Read the model definition and answer for the solid it produces. Units are mm, in the model's axes. A direction names the side the tool comes from. Coordinates: 2 decimals unless noted, no trailing zeros. Loops run counter-clockwise (first coordinate to the right, second up) from the corner with the lowest first, then second, coordinate; pieces in that order, holes last.
Q1. Section B-B (z = 3.9) is taken. Count the separate pieces of the cut face and the enclosed holes in it, then the cut area to 3 significant figures.
Q2. Section A-A (y = 0) is taken. Give the vertices of the cut face in (x, z), then the cut area to 3 significant figures.
Q3. Section C-C (x = 35) is taken. Give the vertices of the cut face in (y, z).
Q4. Which of the six approach directions +Z, -Z, +X, -X, +Y, -Y give full straight-line access (tool end or side, diameter ignored) to faces 1 (the face through (1, 19, 5)), 2 (the face through (69, -31, 3))?
Q5. The mould has two halves that part along Y. Classify faces 3 (the face through (1, -69.382, 2)), 4 (the face through (-3.37, 104.946, 2.465)), 5 (the face through (1, 19, 0)), 6 (the face through (70.87, -39.84, 2.54)): pulls with the +Y half, pulls with the -Y half, needs draft (parallel to the pull), parting line crosses it, or undercut.
Q6. Straight lines are drawn through the part: line 1 (Y direction, x = 0, z = 2.8); line 2 (X direction, y = -44, z = 4); line 3 (Y direction, x = 28, z = 2.5). For each, find the intervals that lie inside material, in ascending order.
Q7. Section D-D (y = 45.5) is taken. Give the vertices of the cut face in (x, z), then the cut area to 3 significant figures.
Q8. Flat-ended cylindrical pins translate along their axes: P1, Ø1.6, axis at x = 28, y = -28, coming from the +Z side; P2, Ø5, axis at x = 0, y = 102.5, coming from the +Z side; P3, Ø1.1, axis at x = 26, z = 2, coming from the +Y side; P4, Ø1.5, axis at y = -3.5, z = 2.5, coming from the -X side. Find the tip coordinate at first contact, or state that the pin passes through.
from build123d import *

# Parameters (mm, degrees)
BOSS_EXTRU_1_DEPTH      = 5
ESQUISSE2_R             = 1.5
ENL_V_MAT_EXTRU_1_DEPTH = 5
ESQUISSE3_R             = 1
ENL_V_MAT_EXTRU_2_DEPTH = 149.576579581
ENL_V_MAT_EXTRU_3_DEPTH = 149.576579581
ESQUISSE5_W             = 3.649999998
ESQUISSE5_H             = 20
ENL_V_MAT_EXTRU_4_DEPTH = 149.576579581


with BuildPart() as part:
    # Esquisse1 → Boss.-Extru.1 (new body)
    with BuildSketch(Plane.XY):
        with BuildLine():
            Line((78.81072608, -69.38205427), (-78.81072608, -69.38205427))
            ThreePointArc((-78.81072608, -69.38205427), (0, 105), (78.81072608, -69.38205427))
        make_face()
    extrude(amount=BOSS_EXTRU_1_DEPTH)

    # Esquisse2 → Enlèv. mat.-Extru.1 (cut)
    with BuildSketch(Plane.XY.offset(5)):
        with Locations((0, 102.5)):
            Circle(ESQUISSE2_R)
        with Locations((72.478445072, 72.478445072)):
            Circle(ESQUISSE2_R)
        with Locations((-72.478445072, 72.478445072)):
            Circle(ESQUISSE2_R)
    extrude(amount=-ENL_V_MAT_EXTRU_1_DEPTH, mode=Mode.SUBTRACT)

    # Esquisse3 → Enlèv. mat.-Extru.2 (cut, through all)
    with BuildSketch(Plane.XY.offset(5)):
        with Locations((20.000000004, 41.999999998)):
            Circle(ESQUISSE3_R)
        with Locations((-19.999999996, 42.000000002)):
            Circle(ESQUISSE3_R)
        with Locations((-28.000000003, -27.999999997)):
            Circle(ESQUISSE3_R)
        with Locations((27.999999997, -28.000000003)):
            Circle(ESQUISSE3_R)
    extrude(amount=-ENL_V_MAT_EXTRU_2_DEPTH, mode=Mode.SUBTRACT)

    # Esquisse4 → Enlèv. mat.-Extru.3 (cut, through all)
    with BuildSketch(Plane.XY.offset(5)):
        Polygon((58.312515902, -42.91606585), (64.096555924, -28.967772728), (73.721801907, -32.959143392), (67.937761885, -46.907436514), align=None)
    extrude(amount=-ENL_V_MAT_EXTRU_3_DEPTH, mode=Mode.SUBTRACT)

    # Esquisse5 → Enlèv. mat.-Extru.4 (cut, through all)
    with BuildSketch(Plane.XY.offset(5)):
        with Locations((26.425, -3e-09)):
            Rectangle(ESQUISSE5_W, ESQUISSE5_H)
    extrude(amount=-ENL_V_MAT_EXTRU_4_DEPTH, mode=Mode.SUBTRACT)


solid = part.part
Numbers:
1. separate pieces: 1
1. enclosed holes: 9
1. area: 30,500 mm2
2. outline: (-105, 0) - (24.6, 0) - (24.6, 5) - (-105, 5) - close; (28.25, 0) - (105, 0) - (105, 5) - (28.25, 5) - close
2. area: 1,030 mm2
3. outline: (-69.38, 0) - (98.99, 0) - (98.99, 5) - (-69.38, 5) - close
4. face 1: +Z, +X, -X, +Y, -Y
4. face 2: +Z, -Z
5. face 3: pulls with the -Y half
5. face 4: parting line crosses it
5. face 5: needs draft
5. face 6: undercut
6. line 1: y = -69.38 to 101, 104 to 105
6. line 2: x = -95.34 to 60.93, 69.14 to 95.34
6. line 3: y = -69.38 to -29, -27 to -10, 10 to 101.2
7. outline: (-94.63, 0) - (94.63, 0) - (94.63, 5) - (-94.63, 5) - close
7. area: 946 mm2
8. P1: passes through
8. P2: stops at z = 5
8. P3: stops at y = 101.87
8. P4: stops at x = -104.96
